Answer from the drawing. Dimensions are ordinates in mm from the lowest x, y and z of the part. A direction names the side the tool comes from. Give positions to 0.01 mm unless a question says otherwise; leave off trailing zeros. Write each loop counter-clockwise with the first axis right and the second up, starting at its lowest first coordinate (ties: lowest second). Pieces come first, ordered by that corner, then holes. Notation, with made-up numbers: (34.5, 0.25) -> (54.5, 0.25) arc R15 cw to (54.5, 17.25) -> close; hole circle Ø11 at (11, -16.5). An arc over 180 degrees is marked (long way). Use a Markdown table: item, result. Add a question column.
Q1. Section A-A, the plane x = 18.1 is taken. State how many separate pieces and enclosed holes the cut face has, plus the area to 3 significant figures.
Q2. Section B-B, the plane y = 37.5 is taken. Give the vertices of the cut face in (x, z) (1 decimal), plus the area to 3 significant figures.
Q3. Each of these flat-tipped pins is pushed along its axis until it touches: pin 1 Ø3.5 at (x, y) = (33.1, 7.5) entering from +Z; pin 2 Ø4.5 at (x, y) = (33.1, 22.225) entering from +Z (1 decimal); pin 3 Ø6 at (y, z) = (11.11, 14.76) entering from -X; pin 4 Ø4 at (y, z) = (33, 10) entering from +X (1 decimal). Where does it stop, or does it pass through?
Q4. Consider line 1 (X direction, y = 7.5, z = 21.75) (1 decimal). Determine where the line is inside the solid, lowest interval first.
Q5. For the marked faces 1 and 2, determine the directions among +Z, -Z, +X, -X, +Y, -Y from which every point of the face is accessible in a straight line to the end or side of a thin tool.
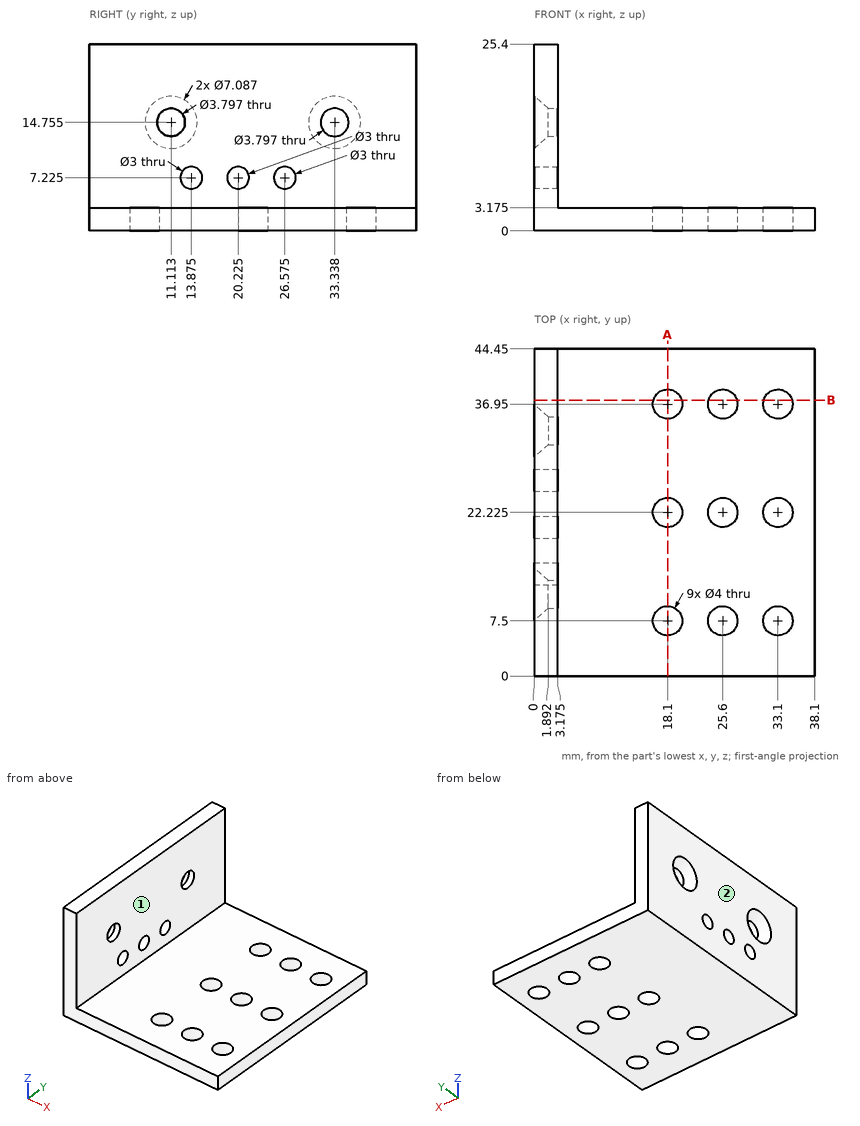
Result set:
| question | item | result |
|---|---|---|
| 1 | separate pieces | 4 |
| 1 | enclosed holes | 0 |
| 1 | area | 103 mm2 |
| 2 | outline | (0, 0) -> (16.2, 0) -> (16.2, 3.2) -> (3.2, 3.2) -> (3.2, 25.4) -> (0, 25.4) -> close; (20, 0) -> (23.7, 0) -> (23.7, 3.2) -> (20, 3.2) -> close; (27.5, 0) -> (31.2, 0) -> (31.2, 3.2) -> (27.5, 3.2) -> close; (35, 0) -> (38.1, 0) -> (38.1, 3.2) -> (35, 3.2) -> close |
| 2 | area | 155 mm2 |
| 3 | pin 1 | passes through |
| 3 | pin 2 | stops at z = 3.2 |
| 3 | pin 3 | stops at x = 0.62 |
| 3 | pin 4 | stops at x = 3.2 |
| 4 | line 1 | x = 0 to 3.2 |
| 5 | face 1 | +Z, +X, +Y, -Y |
| 5 | face 2 | +Z, -Z, -X, +Y, -Y |
